from build123d import *

# Parameters (mm, degrees)
BOSS_EXTRUDE1_DEPTH = 6.35
SKETCH2_R           = 2.4892
CUT_EXTRUDE1_DEPTH  = 7.35
BOSS_EXTRUDE2_DEPTH = 6.35
SKETCH2_4_R         = 2.4892
CUT_EXTRUDE2_DEPTH  = 7.35
FILLET1_R           = 6.35


with BuildPart() as part:
    # Sketch1 → Boss-Extrude1 (new body)
    with BuildSketch(Plane.XY):
        Polygon((0, 156.050081258), (50.8, 228.6), (50.8, 0), (0, 0), align=None)
    extrude(amount=BOSS_EXTRUDE1_DEPTH)

    # Sketch2 → Cut-Extrude1 (cut, through all)
    with BuildSketch(Plane(origin=(0, 0, 0), x_dir=(-1, 0, 0), z_dir=(0, 0, -1))):
        Polygon((-39.347389129, 212.243976613), (-50.8, 228.6), (-50.8, 204.224772149), align=None)
        with Locations((-42.46619935, 194.556324909)):
            Circle(SKETCH2_R)
        with Locations((-35.181778608, 184.153093946)):
            Circle(SKETCH2_R)
        with Locations((-27.897357867, 173.749862984)):
            Circle(SKETCH2_R)
        with Locations((-20.612937125, 163.346632021)):
            Circle(SKETCH2_R)
        with Locations((-13.328516383, 152.943401059)):
            Circle(SKETCH2_R)
        with Locations((-6.044095642, 142.540170097)):
            Circle(SKETCH2_R)
        with Locations((-26.850557567, 127.971328613)):
            Circle(SKETCH2_R)
        with Locations((-19.566136825, 117.568097651)):
            Circle(SKETCH2_R)
        with Locations((-12.281716083, 107.164866688)):
            Circle(SKETCH2_R)
        with Locations((-34.134978308, 138.374559576)):
            Circle(SKETCH2_R)
        with Locations((-41.41939905, 148.777790538)):
            Circle(SKETCH2_R)
        with Locations((-4.997295342, 96.761635726)):
            Circle(SKETCH2_R)
        with Locations((-38.1, 12.7)):
            Circle(SKETCH2_R)
        with Locations((-12.7, 12.7)):
            Circle(SKETCH2_R)
        with Locations((-12.7, 25.4)):
            Circle(SKETCH2_R)
        with Locations((-38.1, 25.4)):
            Circle(SKETCH2_R)
        with Locations((-38.1, 38.1)):
            Circle(SKETCH2_R)
        with Locations((-12.7, 38.1)):
            Circle(SKETCH2_R)
        with Locations((-12.7, 50.8)):
            Circle(SKETCH2_R)
        with Locations((-38.1, 50.8)):
            Circle(SKETCH2_R)
    extrude(amount=-CUT_EXTRUDE1_DEPTH, mode=Mode.SUBTRACT)

    # Sketch3 → Boss-Extrude2 (add)
    with BuildSketch(Plane.XY):
        Polygon((0, 156.050081258), (-33.496818287, 108.211666988), (0, 84.756942318), align=None)
        Polygon((50.8, 204.224772149), (50.8, 140.032902782), (80.960312979, 183.106293646), align=None)
    extrude(amount=BOSS_EXTRUDE2_DEPTH)

    # Sketch2<4> → Cut-Extrude2 (cut, through all)
    with BuildSketch(Plane(origin=(0, 0, 0), x_dir=(-1, 0, 0), z_dir=(0, 0, -1))):
        with Locations((15.809166583, 111.330477209)):
            Circle(SKETCH2_4_R)
        with Locations((8.524745841, 121.733708172)):
            Circle(SKETCH2_4_R)
        with BuildLine():
            ThreePointArc((3.7295251, 132.136939134), (2.487060718, 134.291415158), (0, 134.295112039))
            Line((0, 134.295112039), (0, 129.978766229))
            ThreePointArc((0, 129.978766229), (2.487060718, 129.98246311), (3.7295251, 132.136939134))
        make_face()
        with BuildLine():
            Line((0, 129.978766229), (0, 134.295112039))
            ThreePointArc((0, 134.295112039), (-1.2488749, 132.136939134), (0, 129.978766229))
        make_face()
        with BuildLine():
            ThreePointArc((-46.214619792, 159.181021501), (-48.004425459, 161.569946825), (-50.8, 160.523461508))
            Line((-50.8, 160.523461508), (-50.8, 157.838581493))
            ThreePointArc((-50.8, 157.838581493), (-48.004425459, 156.792096176), (-46.214619792, 159.181021501))
        make_face()
        with BuildLine():
            Line((-50.8, 157.838581493), (-50.8, 160.523461508))
            ThreePointArc((-50.8, 160.523461508), (-51.193019792, 159.181021501), (-50.8, 157.838581493))
        make_face()
        with Locations((-55.988240533, 169.584252463)):
            Circle(SKETCH2_4_R)
        with Locations((-63.272661275, 179.987483426)):
            Circle(SKETCH2_4_R)
    extrude(amount=-CUT_EXTRUDE2_DEPTH, mode=Mode.SUBTRACT)

    # Fillet1
    fillet1_edges = [part.edges().sort_by_distance(p)[0] for p in [
        (-33.496818287, 108.211666988, 3.175),
        (0, 84.756942318, 3.175),
        (50.8, 140.032902782, 3.175),
        (80.960312979, 183.106293646, 3.175),
        (39.347389129, 212.243976613, 3.175),
        (50.8, 0, 3.175),
        (0, 0, 3.175),
    ]]
    fillet(fillet1_edges, radius=FILLET1_R)


solid = part.part
Model file for the job. Use its own axes, mm. Give positions to 0.01 mm unless a question says otherwise; leave off trailing zeros. Order: outer loops, then holes, each group sorted by start corner. A loop starts at its lowest first (then second) coordinate and runs counter-clockwise, first axis right, second up. Notation, with made-up numbers: M 22,5 L 67,5 A8 cw 67,17 Z; hole C 33,58.5 d11. An arc over 180 degrees is marked long. Put each result on its own line as item: value. Start each with the question number.
(1) Drill centre lines: L1, parallel to Y at x = 19.5, z = 3.5; L2, parallel to Y at x = 38.1, z = 1.75; L3, parallel to Y at x = 26.5, z = 3.5. Where is each one in solid material? Low to high. Write a range as [from, to].
(2) Pin check, flat tips, straight feed: pin 1 Ø1 at (x, z) = (58.5, 3) entering from +Y; pin 2 Ø5.5 at (x, y) = (20.61, 163.35) entering from +Z; pin 3 Ø1 at (y, z) = (159.5, 4) entering from -X; pin 4 Ø1.5 at (x, z) = (48.5, 2.5) entering from +Y. Stop position of each tip, or through.
(3) Pull direction Y, two halves, no side cores. Call faces 1 (the face through (-30.92, 108.74, 3.22)), 2 (the face through (22.448, 165.029, 3.131)), 3 (the face through (-15.681, 95.737, 3.131)): released by +Y, released by -Y, zero draft, split by the parting line, or undercut.
(4) Band-saw the part on A-A on y = 50.8. Give the cut face in (x, z).
(5) Band-saw the part on B-B on z = 3. Count the separate pieces of the cut face and the enclosed holes in it, then the cut area to 3 significant figures.
Results below:
1. L1: y = [0, 115.08], [120.06, 161.12], [165.57, 183.9]
1. L2: y = [0, 10.21], [15.19, 22.91], [27.89, 35.61], [40.59, 48.31], [53.29, 209.1]
1. L3: y = [0, 125.51], [130.44, 171.69], [175.81, 193.9]
2. pin 1: stops at y = 199.18
2. pin 2: stops at z = 6.35
2. pin 3: stops at x = 2.07
2. pin 4: stops at y = 206.36
3. face 1: split by the parting line
3. face 2: undercut
3. face 3: released by -Y
4. outline: M 0,0 L 10.21,0 L 10.21,6.35 L 0,6.35 Z; M 15.19,0 L 35.61,0 L 35.61,6.35 L 15.19,6.35 Z; M 40.59,0 L 50.8,0 L 50.8,6.35 L 40.59,6.35 Z
5. separate pieces: 1
5. enclosed holes: 26
5. area: 11,200 mm2
